Design review of the part built by this model. Coordinates are the model's own, in mm. A direction names the side the tool comes from. Give positions to 0.01 mm unless a question says otherwise; leave off trailing zeros. Loops run counter-clockwise (first coordinate to the right, second up) from the corner with the lowest first, then second, coordinate; pieces in that order, holes last. Notation, with made-up numbers: M 77.25,34.5 L 97.25,34.5 A6 ccw 97.25,38.5 Z; hole C -6,39 d5. An arc over 180 degrees is marked long. Use one line per item in the form item = value. Start each with the question number.
from build123d import *

# Parameters (mm, degrees)
F0_W     = 380
F0_H     = 33.5
F1_DEPTH = 1000
F3_DEPTH = 25
F4_R     = 4
F5_DEPTH = 15


# Not quite as in the source:
# - a feature names something its author has since deleted; it is built from what else it names


with BuildPart() as f1:
    # F0 (on Right) → F1 (new body, symmetric)
    with BuildSketch(Plane.YZ):
        with Locations((0, 16.75)):
            Rectangle(F0_W, F0_H)
    extrude(amount=F1_DEPTH, both=True)

    # F2 (on face) → F3 (join)
    with BuildSketch(Plane(origin=(0, 0, 0), x_dir=(1, 0, 0), z_dir=(0, 0, -1))):
        with BuildLine():
            ThreePointArc((-790, -190), (-655.6497115746, -134.3502884254), (-600, 0))
            ThreePointArc((-600, 0), (-655.6497118153, 134.3502886662), (-790.0000006809, 190))
            ThreePointArc((-790.0000006809, 190), (-980, -3.405e-07), (-790, -190))
        make_face()
        with BuildLine():
            ThreePointArc((190, 0), (134.350288533, 134.3502883179), (3.042e-07, 190))
            ThreePointArc((3.042e-07, 190), (-190, 1.521e-07), (0, -190))
            ThreePointArc((0, -190), (134.3502884254, -134.3502884254), (190, 0))
        make_face()
        with BuildLine():
            ThreePointArc((980, 0), (924.3502884254, 134.3502884254), (790, 190))
            ThreePointArc((790, 190), (600, 0), (790, -190))
            ThreePointArc((790, -190), (924.3502884254, -134.3502884254), (980, 0))
        make_face()
    extrude(amount=F3_DEPTH)

    # F4 (on face) → F5 (join)
    with BuildSketch(Plane(origin=(0, 0, 0), x_dir=(1, 0, 0), z_dir=(0, 0, -1))):
        Polygon((-990, 190), (-1000, 190), (-1000, 70), (-1000, -190), (-990, -190), (-990, -140), (-990, 140), align=None)
        Polygon((-910, 190), (-990, 190), (-990, 140), (-935.7230966807, 140), (-910, 166.1522239447), align=None)
        with Locations((-980, 180)):
            Circle(F4_R, mode=Mode.SUBTRACT)
        with Locations((-920, 180)):
            Circle(F4_R, mode=Mode.SUBTRACT)
        Polygon((-990, -140), (-990, -190), (-910, -190), (-910, -166.1522239447), (-935.7230966807, -140), align=None)
        with Locations((-980, -180)):
            Circle(F4_R, mode=Mode.SUBTRACT)
        with Locations((-920, -180)):
            Circle(F4_R, mode=Mode.SUBTRACT)
        Polygon((-590, 190), (-670, 190), (-670, 166.1522239447), (-644.2769033193, 140), (-590, 140), align=None)
        with Locations((-660, 180)):
            Circle(F4_R, mode=Mode.SUBTRACT)
        with Locations((-600, 180)):
            Circle(F4_R, mode=Mode.SUBTRACT)
        Polygon((-670, -166.1522239447), (-670, -190), (-590, -190), (-590, -140), (-644.2769033193, -140), align=None)
        with Locations((-660, -180)):
            Circle(F4_R, mode=Mode.SUBTRACT)
        with Locations((-600, -180)):
            Circle(F4_R, mode=Mode.SUBTRACT)
        Polygon((-120, 190), (-200, 190), (-200, 140), (-145.7230966807, 140), (-120, 166.1522239447), align=None)
        with Locations((-190, 180)):
            Circle(F4_R, mode=Mode.SUBTRACT)
        with Locations((-130, 180)):
            Circle(F4_R, mode=Mode.SUBTRACT)
        Polygon((-200, -140), (-200, -190), (-120, -190), (-120, -166.1522239447), (-145.7230966807, -140), align=None)
        with Locations((-190, -180)):
            Circle(F4_R, mode=Mode.SUBTRACT)
        with Locations((-130, -180)):
            Circle(F4_R, mode=Mode.SUBTRACT)
        Polygon((200, 190), (120, 190), (120, 166.1522239447), (145.7230966807, 140), (200, 140), align=None)
        with Locations((130, 180)):
            Circle(F4_R, mode=Mode.SUBTRACT)
        with Locations((190, 180)):
            Circle(F4_R, mode=Mode.SUBTRACT)
        Polygon((120, -166.1522239447), (120, -190), (200, -190), (200, -140), (145.7230966807, -140), align=None)
        with Locations((130, -180)):
            Circle(F4_R, mode=Mode.SUBTRACT)
        with Locations((190, -180)):
            Circle(F4_R, mode=Mode.SUBTRACT)
        Polygon((590, -140), (590, -190), (670, -190), (670, -166.1522239447), (644.2769033193, -140), align=None)
        with Locations((600, -180)):
            Circle(F4_R, mode=Mode.SUBTRACT)
        with Locations((660, -180)):
            Circle(F4_R, mode=Mode.SUBTRACT)
        Polygon((670, 190), (590, 190), (590, 140), (644.2769033193, 140), (670, 166.1522239447), align=None)
        with Locations((600, 180)):
            Circle(F4_R, mode=Mode.SUBTRACT)
        with Locations((660, 180)):
            Circle(F4_R, mode=Mode.SUBTRACT)
        Polygon((910, -166.1522239447), (910, -190), (990, -190), (990, -140), (935.7230966807, -140), align=None)
        with Locations((920, -180)):
            Circle(F4_R, mode=Mode.SUBTRACT)
        with Locations((980, -180)):
            Circle(F4_R, mode=Mode.SUBTRACT)
        Polygon((990, 190), (910, 190), (910, 166.1522239447), (935.7230966807, 140), (990, 140), align=None)
        with Locations((920, 180)):
            Circle(F4_R, mode=Mode.SUBTRACT)
        with Locations((980, 180)):
            Circle(F4_R, mode=Mode.SUBTRACT)
        Polygon((990, -140), (990, -190), (1000, -190), (1000, -70), (1000, 70), (1000, 190), (990, 190), (990, 140), align=None)
    extrude(amount=F5_DEPTH)


solid = f1.part
Q1. Take a section at B-B on y = -90.5. Give the boundary of the cut face in (x, z), plus the area to 3 significant figures.
Q2. For faces 5 (the flat face through (-631, -165, -15)), 6 (the cylindrical face through (-115.61, -150.78, -12.32)), 7 (the flat face through (-161, 165, -15)), list the 3-axis set-ups (+Z, -Z, +X, -X, +Y, -Y) from which the entire face can be reached by the end or side of a thin tool; tool diameter is ignored.
Q3. Clearance check with flat-ended pins moving along their axes: pin 1 Ø15 at (x, y) = (-153, 170.5) entering from -Z; pin 2 Ø4 at (y, z) = (-12.5, -17.5) entering from +X; pin 3 Ø7 at (x, y) = (-980, 180) entering from -Z. State where each tip first meets the part, or that it passes through.
Q4. Take a section at A-A on y = 0. Give the boundary of the cut face in (x, z).
Q5. Wall thickness on probe 1 along X at (y, z) = (-11, -5.5); probe 2 along X at (y, z) = (-169, -22); probe 3 along Y at (x, z) = (-130, -11): over which ranges is each line inside the solid? List them lowest first.
Q6. The part is to be moulded in two halves that separate along Y. For faces 1 (the flat face through (-3, -3, -25)), 2 (the cylindrical face through (-978.383, 24.734, -12.325)), 3 (the flat face through (14, -190, 15)), 4 (the flat face through (-14, 190, 15)), say which applies: pulls with the +Y half, pulls with the -Y half, needs draft (parallel to the pull), parting line crosses it, or undercut.
Response values:
q1.outline = M -1000,-15 L -990,-15 L -990,0 L -957.06,0 L -957.06,-25 L -622.94,-25 L -622.94,0 L -167.06,0 L -167.06,-25 L 167.06,-25 L 167.06,0 L 622.94,0 L 622.94,-25 L 957.06,-25 L 957.06,0 L 990,0 L 990,-15 L 1000,-15 L 1000,33.5 L -1000,33.5 Z
q1.area = 92,400 mm^2
q2.face_5 = -Z, -Y
q2.face_6 = -Z
q2.face_7 = -Z, +Y
q3.pin_1 = -15
q3.pin_2 = 979.71
q3.pin_3 = 0
q4.outline = M -1000,-15 L -990,-15 L -990,0 L -980,0 L -980,-25 L -600,-25 L -600,0 L -190,0 L -190,-25 L 190,-25 L 190,0 L 600,0 L 600,-25 L 980,-25 L 980,0 L 990,0 L 990,-15 L 1000,-15 L 1000,33.5 L -1000,33.5 Z
q5.probe_1 = -1000 to -990, -979.68 to -600.32, -189.68 to 189.68, 600.32 to 979.68, 990 to 1000
q5.probe_2 = -876.83 to -703.17, -86.83 to 86.83, 703.17 to 876.83
q5.probe_3 = -190 to -184, -176 to -155.99, -138.56 to 138.56, 155.99 to 176, 184 to 190
q6.face_1 = needs draft
q6.face_2 = undercut
q6.face_3 = pulls with the -Y half
q6.face_4 = pulls with the +Y half
